```python
from build123d import *

# Parameters (mm, degrees)
SKETCH_1_W          = 12
SKETCH_1_H          = 12
SKETCH_1_W_2        = 10
SKETCH_1_H_2        = 10
EXTRUDE_1_DEPTH     = 10
SKETCH_2_W          = 12
SKETCH_2_H          = 12
EXTRUDE_2_DEPTH     = 5
SKETCH_3_R          = 1
CUT_EXTRUDE_3_DEPTH = 12


with BuildPart() as part:
    # 草图1 → 凸台-拉伸1 (new body)
    with BuildSketch(Plane.XY):
        with Locations((6, 6)):
            Rectangle(SKETCH_1_W, SKETCH_1_H)
        with Locations((6, 6)):
            Rectangle(SKETCH_1_W_2, SKETCH_1_H_2, mode=Mode.SUBTRACT)
    extrude(amount=EXTRUDE_1_DEPTH)

    # 草图2 → 凸台-拉伸2 (add)
    with BuildSketch(Plane.XY.offset(10)):
        with Locations((6, 6)):
            Rectangle(SKETCH_2_W, SKETCH_2_H)
    extrude(amount=EXTRUDE_2_DEPTH)

    # 草图3 → 切除-拉伸3 (cut)
    with BuildSketch(Plane(origin=(0, 0, 0), x_dir=(-1, 0, 0), z_dir=(0, -1, 0))):
        with Locations(Location((-6, -12.5, 0), (0, 0, 90))):
            Circle(SKETCH_3_R)
    extrude(amount=-CUT_EXTRUDE_3_DEPTH, mode=Mode.SUBTRACT)


solid = part.part
```
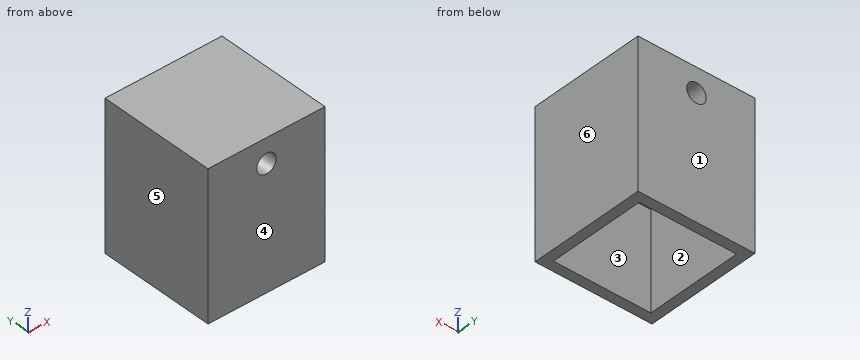
The listing builds one solid part. Answer for the finished solid, in the listing's coordinates (mm). Face numbers are marked on the shaded views. A direction names the side the tool comes from. Give positions to 0.01 mm unless a question says otherwise; leave off trailing zeros. Write each loop counter-clockwise with the first axis right and the second up, starting at its lowest first coordinate (ties: lowest second). Pieces come first, ordered by that corner, then holes. Notation, with made-up numbers: M -33,86 L -2,86 A16 ccw -2,92 Z; hole C -23.5,31 d10. An arc over 180 degrees is marked long. Write each question's results on one line, items separated by ' | '.
Q1. Section C-C, the plane z = 12.5 is taken. Write down the section's boundary in (x, y).
Output values:
outline: M 0,0 L 5,0 L 5,12 L 0,12 Z; M 7,0 L 12,0 L 12,12 L 7,12 Z
Q2. For a pull along X with two mould halves and no side action, classify the marked faces 3, 4, 5 and 6 as released by +X, released by -X, zero draft, split by the parting line, or undercut.
Output values:
face 3: undercut | face 4: zero draft | face 5: released by -X | face 6: released by +X
Q3. Section D-D, the plane y = 8 is taken. Write down the section's boundary in (x, z), then the cut area to 3 significant figures.
Output values:
outline: M 0,0 L 1,0 L 1,10 L 11,10 L 11,0 L 12,0 L 12,15 L 0,15 Z; hole C 6,12.5 d2 | area: 76.9 mm2
Q4. A tool of negligible diameter and unlimited length cuts with its end or side. For the marked faces 1 and 2, from which of +Z, -Z, +X, -X, +Y, -Y can it reach the whole face along a straight path? Write none if from no direction.
Output values:
face 1: +Z, -Z, +X, -X, +Y | face 2: -Z
Q5. Section B-B, the plane x = 6 is taken. Write down the section's boundary in (y, z).
Output values:
outline: M 0,0 L 1,0 L 1,10 L 11,10 L 11,0 L 12,0 L 12,11.5 L 0,11.5 Z; M 0,13.5 L 12,13.5 L 12,15 L 0,15 Z
Q6. Consider L1, parallel to X at y = 7.75, z = 12.5; L2, parallel to Y at x = 6.75, z = 3. Determine where each line is inside the solid, lowest interval first. Write a range as from..to.
Output values:
L1: 0..5, 7..12 | L2: 0..1, 11..12
Q7. Section A-A, the plane z = 3.75 is taken. Write down the section's boundary in (x, y), then the cut area to 3 significant figures.
Output values:
outline: M 0,0 L 12,0 L 12,12 L 0,12 Z; hole M 1,1 L 11,1 L 11,11 L 1,11 Z | area: 44.0 mm2
